from build123d import *

# Parameters (mm, degrees)
F0_W     = 60
F0_H     = 40
F0_W_2   = 54
F0_H_2   = 34
F1_DEPTH = 555
F3_DEPTH = 60
F4_DEPTH = 60


with BuildPart() as f1:
    # F0 (on Top) → F1 (new body)
    with BuildSketch(Plane.XY):
        Rectangle(F0_W, F0_H)
        Rectangle(F0_W_2, F0_H_2, mode=Mode.SUBTRACT)
    extrude(amount=F1_DEPTH)

    # F2 (on face) → F3 (cut)
    with BuildSketch(Plane.YZ.offset(30)):
        Polygon((20, 555), (-17, 555), (20, 518), align=None)
        Polygon((-17, 0), (20, 0), (20, 37), align=None)
    extrude(amount=-F3_DEPTH, mode=Mode.SUBTRACT)

    # F2 (on face) → F4 (cut)
    with BuildSketch(Plane.YZ.offset(30)):
        Polygon((20, 0), (20, 37), (-17, 0), align=None)
    extrude(amount=-F4_DEPTH, mode=Mode.SUBTRACT)


solid = f1.part
The model under review builds one solid part; all positions refer to its coordinate system, in mm. A direction names the side the tool comes from. Round coordinates to 2 decimals unless told otherwise and drop trailing zeros. Write each loop counter-clockwise with the first axis right and the second up, starting at its lowest first coordinate (ties: lowest second). Pieces come first, ordered by that corner, then holes. Notation, with made-up numbers: (-33, 62) -> (15, 62) arc R11 ccw to (15, 82) -> close; hole circle Ø11 at (18.5, -31.75). An arc over 180 degrees is marked (long way). Answer as a JSON object with one key per item and string values.
1. We need section B-B on x = 10. State the section outline as (y, z) points.
Results found:
{"outline": "(-20, 0) -> (-17, 0) -> (-17, 555) -> (-20, 555) -> close; (17, 34) -> (20, 37) -> (20, 518) -> (17, 521) -> close"}
2. The part is to be moulded in two halves that separate along Y. For faces 1 (the face through (-30, 0, 274)), 2 (the face through (0, -17, 274)), 3 (the face through (27, 0, 274)), 4 (the face through (0, 18, 35)), say which applies: pulls with the +Y half, pulls with the -Y half, needs draft (parallel to the pull), parting line crosses it, or undercut.
Results found:
{"face 1": "needs draft", "face 2": "undercut", "face 3": "undercut", "face 4": "pulls with the +Y half"}
3. We need section A-A on y = -10. State the section outline as (x, z) points, and give its area (3 significant figures).
Results found:
{"outline": "(-30, 7) -> (-27, 7) -> (-27, 548) -> (-30, 548) -> close; (27, 7) -> (30, 7) -> (30, 548) -> (27, 548) -> close", "area": "3,250 mm^2"}
4. Machinability: for faces 5 (the face through (0, 20, 274)), 6 (the face through (0, 17, 274)), which of the approach directions +Z, -Z, +X, -X, +Y, -Y give a long, thin tool a straight path to every point of the face, cutting with its end or side? Answer none if there is none.
Results found:
{"face 5": "+Z, -Z, +X, -X, +Y", "face 6": "+Z, -Z"}
5. We need section C-C on z = 77.5. State the section outline as (x, y) points, and give its area (3 significant figures).
Results found:
{"outline": "(-30, -20) -> (30, -20) -> (30, 20) -> (-30, 20) -> close; hole (-27, -17) -> (27, -17) -> (27, 17) -> (-27, 17) -> close", "area": "564 mm^2"}
6. To check wall thickness, follow line 1 along X through (y, z) = (-11.5, 314); line 2 along Y through (x, z) = (6.5, 237); line 3 along Z through (x, y) = (24, 18). State the ranges of each line that lie inside material, in increasing order.
Results found:
{"line 1": "x = -30 to -27, 27 to 30", "line 2": "y = -20 to -17, 17 to 20", "line 3": "z = 35 to 520"}
